```python
from build123d import *

# Parameters (mm, degrees)
F0_W          = 332.74
F0_H          = 215.9
F0_W_2        = 294.64
F0_H_2        = 177.8
F1_DEPTH      = 9.525
F1_DEPTH_BACK = 9.525
F2_W          = 307.34
F2_H          = 190.5
F3_DEPTH      = 0.0625
F3_DEPTH_BACK = 1.6002


# Not quite as in the source:
# - a pattern or mirror of a feature is missing from the dataset's text; its kind, count and spacing are read off the source's solid


with BuildPart() as f1:
    # F0 (on Front) → F1 (new body, two sides)
    with BuildSketch(Plane.XZ) as f1_sk:
        Rectangle(F0_W, F0_H)
        Rectangle(F0_W_2, F0_H_2, mode=Mode.SUBTRACT)
    extrude(amount=F1_DEPTH)
    extrude(f1_sk.sketch, amount=-F1_DEPTH_BACK)

    # F2 (on Front) → F3 (cut, two sides)
    with BuildSketch(Plane.XZ) as f3_sk:
        Rectangle(F2_W, F2_H)
    f3 = extrude(amount=-F3_DEPTH, mode=Mode.SUBTRACT) + extrude(f3_sk.sketch, amount=F3_DEPTH_BACK, mode=Mode.SUBTRACT)

    # F3_copies: F3 across plane
    add(f3.mirror(Plane.ZX.offset(-0.00635)), mode=Mode.SUBTRACT)


solid = f1.part
```
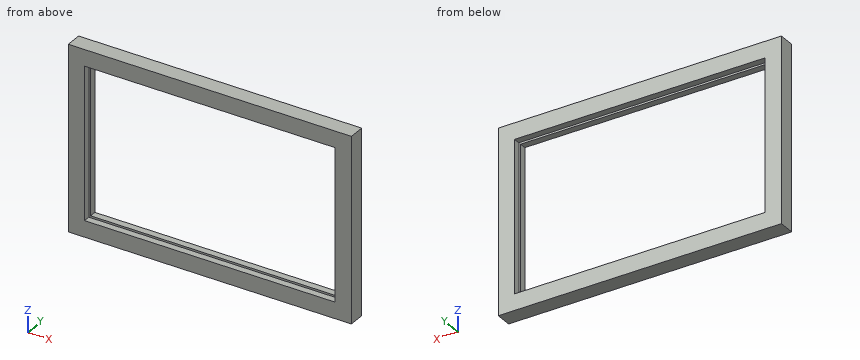
Can you work these out from the model? Positions are in its coordinate system, mm. Round coordinates to 2 decimals unless told otherwise and drop trailing zeros. Order: outer loops, then holes, each group sorted by start corner. A loop starts at its lowest first (then second) coordinate and runs counter-clockwise, first axis right, second up. Notation, with made-up numbers: (60, 50.25) -> (82, 50.25) arc R24 cw to (82, 71.25) -> close; hole circle Ø6 at (76.25, 5.25). An arc over 180 degrees is marked (long way). Return JSON: item names as keys, results as strings. Group by question number.
1. I need wall thicknesses on line 1 (Z direction, x = 32.5, y = -8.5); line 2 (X direction, y = 4.75, z = -49.5); line 3 (X direction, y = -1.5, z = -53.5). Which ranges of each line are inside material? Lowest first, please. Write a range as [from, to].
2. If we section it at B-B, the plane z = -42: Write out the boundary of the cut face in (x, y) (1 decimal), then the cut area to 3 significant figures.
3. If we section it at C-C, the plane y = -5.5: Write out the boundary of the cut face in (x, z).
Output values:
{
 "1": {"line 1": "[-107.95, -88.9], [88.9, 107.95]", "line 2": "[-166.37, -147.32], [147.32, 166.37]", "line 3": "[-166.37, -153.67], [153.67, 166.37]"},
 "2": {"outline": "(-166.4, -9.5) -> (-147.3, -9.5) -> (-147.3, -1.6) -> (-153.7, -1.6) -> (-153.7, 1.6) -> (-147.3, 1.6) -> (-147.3, 9.5) -> (-166.4, 9.5) -> close; (147.3, -9.5) -> (166.4, -9.5) -> (166.4, 9.5) -> (147.3, 9.5) -> (147.3, 1.6) -> (153.7, 1.6) -> (153.7, -1.6) -> (147.3, -1.6) -> close", "area": "685 mm²"},
 "3": {"outline": "(-166.37, -107.95) -> (166.37, -107.95) -> (166.37, 107.95) -> (-166.37, 107.95) -> close; hole (-147.32, -88.9) -> (147.32, -88.9) -> (147.32, 88.9) -> (-147.32, 88.9) -> close"}
}
